from build123d import *

# Parameters (mm, degrees)
F0_R          = 23.1250603282
F1_DEPTH      = 711.2
F2_R          = 44.8716829259
F3_DEPTH      = 609.6
F3_DEPTH_BACK = 609.6
F4_R          = 37.4216193061
F5_DEPTH      = 881.38
F8_R          = 35.8974591154
F9_DEPTH      = 820.42


# Not quite as in the source:
# - a feature of the source that left no trace in its solid (it failed there, or was rolled back) is left out


with BuildPart() as f1:
    # F0 (on Top) → F1 (new body)
    with BuildSketch(Plane.XY):
        Circle(F0_R)
    extrude(amount=F1_DEPTH)

    # F2 (on Right) → F3 (join, two sides)
    with BuildSketch(Plane.YZ) as f3_sk:
        Circle(F2_R)
    extrude(amount=F3_DEPTH)
    extrude(f3_sk.sketch, amount=-F3_DEPTH_BACK)

    # F4 (on Top) → F5 (join)
    with BuildSketch(Plane.XY):
        Circle(F4_R)
    extrude(amount=F5_DEPTH)

    # F8 (on Right) → F9 (join)
    with BuildSketch(Plane.YZ):
        with Locations((0, 320.2763795853)):
            Circle(F8_R)
    extrude(amount=F9_DEPTH)


solid = f1.part
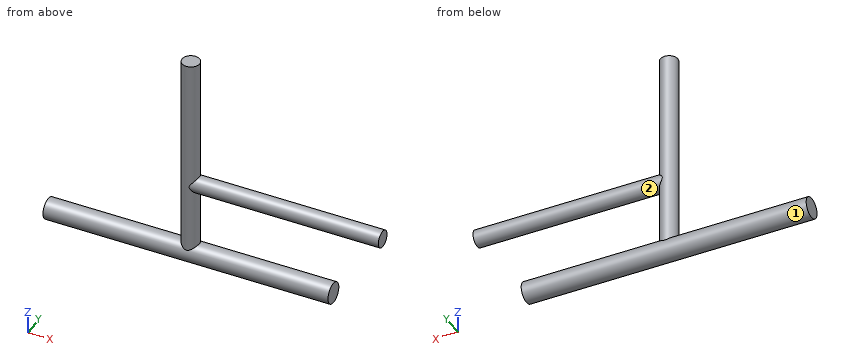
CAD build for the part. Positions are in the model's coordinates, mm. Face numbers are marked on the shaded views. A direction names the side the tool comes from. Give positions to 0.01 mm unless a question says otherwise; leave off trailing zeros. Loops run counter-clockwise (first coordinate to the right, second up) from the corner with the lowest first, then second, coordinate; pieces in that order, holes last. Notation, with made-up numbers: M 24,57.25 L 72,57.25 A31 cw 72,92.25 Z; hole C 89.5,10 d6. An arc over 180 degrees is marked long. Answer in a Markdown table with one row per item. Add a question column.
Item 1: Band-saw the part on D-D on x = -417. Give the cut face in (y, z), then the cut area to 3 significant figures.
Item 2: Band-saw the part on B-B on x = 404. Give the cut face in (y, z).
Item 3: Band-saw the part on C-C on z = 0. Give the cut face in (x, y), then the cut area to 3 significant figures.
Item 4: Drop flat-ended pins along their axis: P1, Ø8, axis at x = 298, y = 22, coming from the -Z side; P2, Ø12, axis at x = -326, y = 7, coming from the +Z side; P3, Ø6, axis at y = 11, z = 595, coming from the +X side. Give the stop position or say it passes through.
Item 5: Band-saw the part on A-A on y = 0. Give the cut face in (x, z).
Item 6: Tool access for the marked faces 1 and 2: list every direction of +Z, -Z, +X, -X, +Y, -Y with a clear straight run to the whole face (end or side of a thin tool).
Item 7: Probe probe 1 along Z at (x, y) = (330, 1.5); probe 2 along Z at (x, y) = (139, 22); probe 3 along X at (y, z) = (-1, 78). List the from-to ranges inside material, lowest first.
Reply:
| question | item | result |
|---|---|---|
| 1 | outline | C 0,0 d89.74 |
| 1 | area | 6,330 mm^2 |
| 2 | outline | C 0,0 d89.74; C 0,320.28 d71.79 |
| 3 | outline | M -609.6,-44.87 L 609.6,-44.87 L 609.6,44.87 L -609.6,44.87 Z |
| 3 | area | 109,000 mm^2 |
| 4 | P1 | stops at z = -41.1 |
| 4 | P2 | stops at z = 44.86 |
| 4 | P3 | stops at x = 36.56 |
| 5 | outline | M -609.6,-44.87 L 609.6,-44.87 L 609.6,44.87 L 37.42,44.87 L 37.42,284.38 L 820.42,284.38 L 820.42,356.17 L 37.42,356.17 L 37.42,881.38 L -37.42,881.38 L -37.42,44.87 L -609.6,44.87 Z |
| 6 | face 1 | none |
| 6 | face 2 | +X |
| 7 | probe 1 | z = -44.85 to 44.85, 284.41 to 356.14 |
| 7 | probe 2 | z = -39.11 to 39.11, 291.91 to 348.64 |
| 7 | probe 3 | x = -37.41 to 37.41 |
